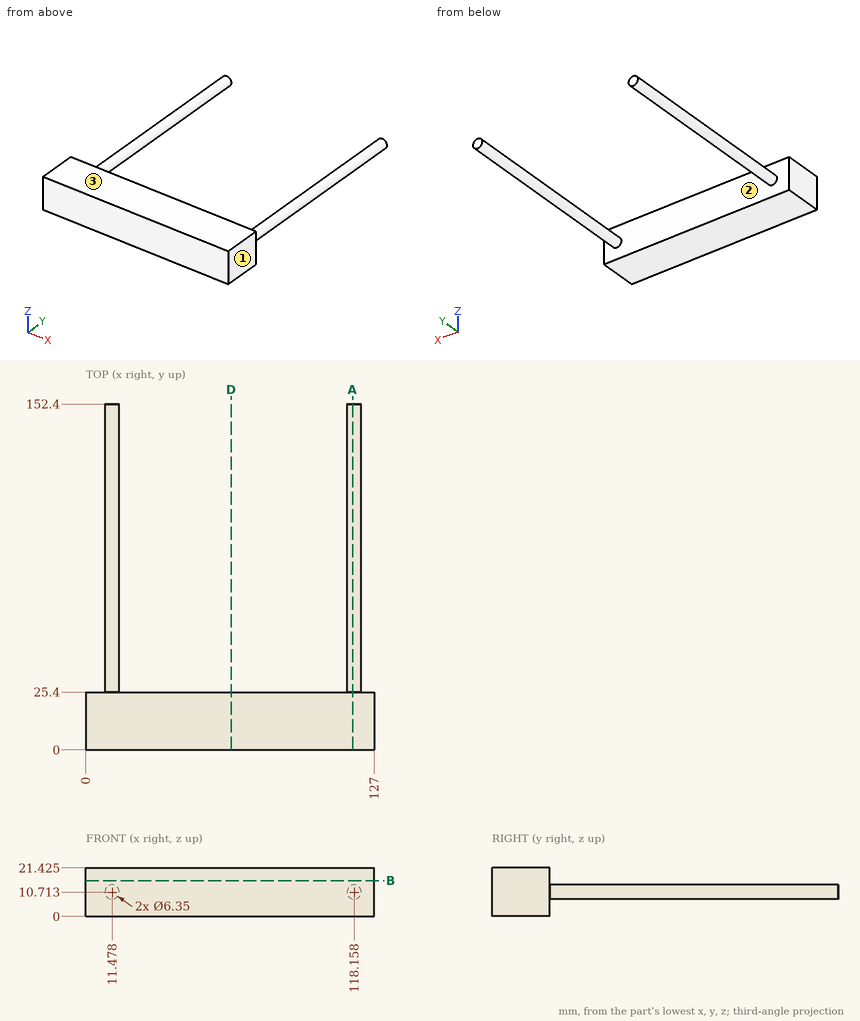
Design review of the part shown in the three views and the two pictorial views. Dimensions are in mm from the part's minimum x, y and z. Coordinates: 2 decimals unless noted, no trailing zeros. Order: outer loops, then holes, each group sorted by start corner. A loop starts at its lowest first (then second) coordinate and runs counter-clockwise, first axis right, second up.
1) Take a section at A-A, the plane x = 117.5. Give the boundary of the cut face in (y, z) (1 decimal).
2) Wall thickness on line 1 along Y through (x, z) = (59, 11.5); line 2 along X through (y, z) = (81.5, 9.5) (1 decimal); line 3 along X through (y, z) = (106, 8) (1 decimal): over which ranges is each line inside the solid? List them lowest first.
3) Take a section at D-D, the plane x = 64. Give the boundary of the cut face in (y, z) (1 decimal).
4) Take a section at B-B, the plane z = 15.75. Give the boundary of the cut face in (x, y).
5) Mouldability with a two-part tool opening along X and no side actions: class the marked faces 1, 2 and 3 as +X half, -X half, draft (parallel to the pull), parting line (faces both ways), or undercut.
6) Clearance check with flat-ended pins moving along their axes: pin 1 (8 mm diameter, centred on y = 132, z = 7, fed in from -X); pin 2 (1.5 mm diameter, centred on y = 131.5, z = 16.5, fed in from -X). State where each tip first meets the part, or that it passes through.
Returned:
1. outline: (0, 0) - (25.4, 0) - (25.4, 7.6) - (152.4, 7.6) - (152.4, 13.8) - (25.4, 13.8) - (25.4, 21.4) - (0, 21.4) - close
2. line 1: y = 0 to 25.4
2. line 2: x = 8.5 to 14.4, 115.2 to 121.1
2. line 3: x = 9.8 to 13.1, 116.5 to 119.8
3. outline: (0, 0) - (25.4, 0) - (25.4, 21.4) - (0, 21.4) - close
4. outline: (0, 0) - (127, 0) - (127, 25.4) - (0, 25.4) - close
5. face 1: +X half
5. face 2: undercut
5. face 3: draft
6. pin 1: stops at x = 8.3
6. pin 2: passes through
